Source: three-view drawing plus pictorial views. Frame: mm from the lowest corner of the part. A direction names the side the tool comes from. Give positions to 0.01 mm unless a question says otherwise; leave off trailing zeros. Order: outer loops, then holes, each group sorted by start corner. A loop starts at its lowest first (then second) coordinate and runs counter-clockwise, first axis right, second up. Notation, with made-up numbers: (72.25, 25.5) -> (117.25, 25.5) arc R34 ccw to (117.25, 62.5) -> close; hole circle Ø10 at (80, 49). An arc over 180 degrees is marked (long way). One line per question, with ' | ' between items.
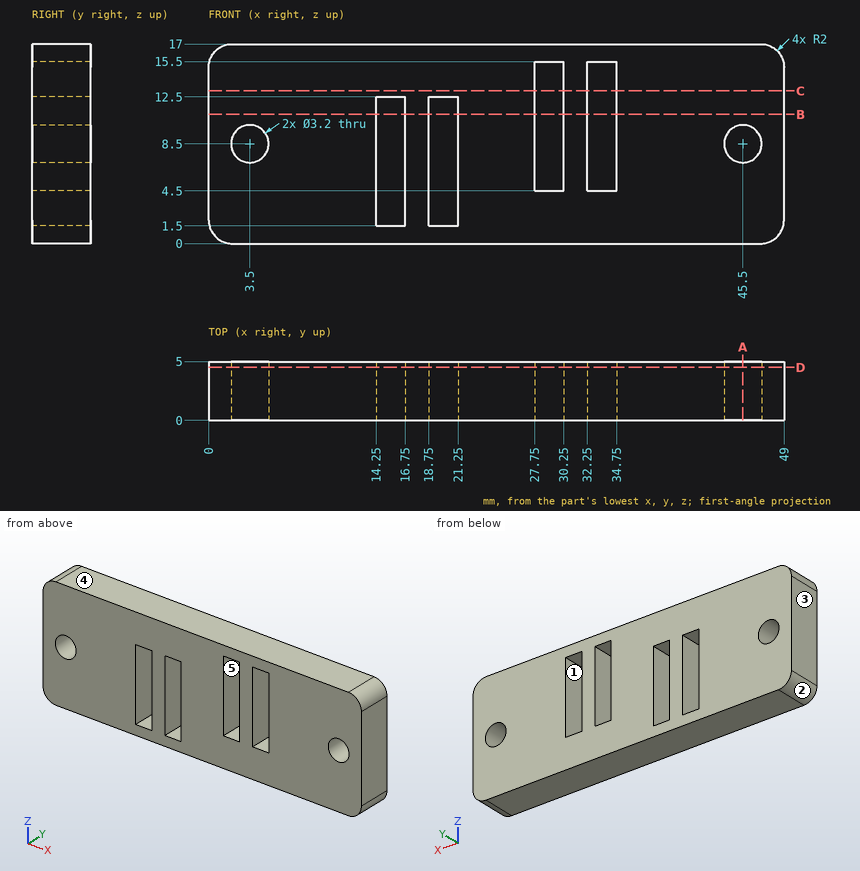
1) Section A-A on x = 45.5. Return loops of the section in (y, z), plus the area to 3 significant figures.
Check result:
outline: (0, 0) -> (5, 0) -> (5, 6.9) -> (0, 6.9) -> close; (0, 10.1) -> (5, 10.1) -> (5, 17) -> (0, 17) -> close | area: 69.0 mm^2
2) Section B-B on z = 11. Return loops of the section in (x, y).
Check result:
outline: (0, 0) -> (14.25, 0) -> (14.25, 5) -> (0, 5) -> close; (16.75, 0) -> (18.75, 0) -> (18.75, 5) -> (16.75, 5) -> close; (21.25, 0) -> (27.75, 0) -> (27.75, 5) -> (21.25, 5) -> close; (30.25, 0) -> (32.25, 0) -> (32.25, 5) -> (30.25, 5) -> close; (34.75, 0) -> (49, 0) -> (49, 5) -> (34.75, 5) -> close
3) Material intervals for probe 1 along X at (y, z) = (3.3, 13); probe 2 along Z at (x, y) = (34.5, 2.4); probe 3 along X at (y, z) = (1.55, 6), sorted ascending. Write a range as from..to.
Check result:
probe 1: x = 0..27.75, 30.25..32.25, 34.75..49 | probe 2: z = 0..4.5, 15.5..17 | probe 3: x = 0..14.25, 16.75..18.75, 21.25..27.75, 30.25..32.25, 34.75..49
4) Section C-C on z = 13. Return loops of the section in (x, y).
Check result:
outline: (0, 0) -> (27.75, 0) -> (27.75, 5) -> (0, 5) -> close; (30.25, 0) -> (32.25, 0) -> (32.25, 5) -> (30.25, 5) -> close; (34.75, 0) -> (49, 0) -> (49, 5) -> (34.75, 5) -> close
5) Set-up query: the marked faces 1 and 2. Return all of +Z, -Z, +X, -X, +Y, -Y with unobstructed straight access to the full face (end or side cutting, diameter ignored); none if empty.
Check result:
face 1: +Y, -Y | face 2: -Z, -X, +Y, -Y
6) Section D-D on y = 4.5. Return loops of the section in (x, z), plus the area to 3 significant figures.
Check result:
outline: (0, 2) arc R2 ccw to (2, 0) -> (47, 0) arc R2 ccw to (49, 2) -> (49, 15) arc R2 ccw to (47, 17) -> (2, 17) arc R2 ccw to (0, 15) -> close; hole circle Ø3.2 at (3.5, 8.5); hole (14.25, 1.5) -> (16.75, 1.5) -> (16.75, 12.5) -> (14.25, 12.5) -> close; hole (18.75, 1.5) -> (21.25, 1.5) -> (21.25, 12.5) -> (18.75, 12.5) -> close; hole (27.75, 4.5) -> (30.25, 4.5) -> (30.25, 15.5) -> (27.75, 15.5) -> close; hole (32.25, 4.5) -> (34.75, 4.5) -> (34.75, 15.5) -> (32.25, 15.5) -> close; hole circle Ø3.2 at (45.5, 8.5) | area: 703 mm^2
7) Pull-direction query (X, two-part tool) for the marked faces 3, 4 and 5; classes: +X half, -X half, draft (parallel to the pull), parting line (faces both ways), or undercut.
Check result:
face 3: -X half | face 4: draft | face 5: undercut
